Check sheet for the modelled part. Datum: model origin and axes. Units: mm. Face numbers are marked on the shaded views. A direction names the side the tool comes from. Coordinates: 2 decimals unless noted, no trailing zeros. Write each loop counter-clockwise with the first axis right and the second up, starting at its lowest first coordinate (ties: lowest second). Pieces come first, ordered by that corner, then holes. Notation, with made-up numbers: M -17,-16.5 L 13,-16.5 A11 ccw 13,3.5 Z; hole C 68.25,-10 d9. An arc over 180 degrees is marked long. Answer as CSV lines item,"result". Start each with the question number.
1) Draft check along Y on the marked faces 6, 7, 8 and 9. Enter one of: +Y half, -Y half, draft (parallel to the pull), parting line (faces both ways), or undercut.
2) Section check A-A (z = 12.5). Record the cut outline in (x, y), and give its area (3 significant figures).
3) Section check D-D (y = 38.25). Record the cut outline in (x, z).
4) Section check C-C (z = 15.75). Record the cut outline in (x, y).
5) Section check B-B (y = 50.25). Record the cut outline in (x, z), and give its area (3 significant figures).
6) Access from +Z, -Z, +X, -X, +Y, -Y to the whole of each face (thin tool, end or side, straight path). Record for the marked faces 1, 2, 3, 4 and 5.
7) Go/stop test with flat-tipped pins: pin 1 Ø6 at (x, y) = (-21.5, 54.5) entering from -Z; pin 2 Ø1.5 at (y, z) = (31.5, 19) entering from +X; pin 3 Ø6 at (x, y) = (-18.5, 10.5) entering from -Z. Record where each tip stops, or that it passes through.
8) Material ranges on L1, parallel to X at y = 38.25, z = 18.25; L2, parallel to X at y = 39, z = 24.25; L3, parallel to Y at x = -17, z = 19.75, recorded low to high. Write a range as [from, to].
from build123d import *

# Parameters (mm, degrees)
SKETCH_1_R          = 5
SKETCH_1_R_2        = 1.5
EXTRUDE_1_DEPTH     = 25
SKETCH_2_R          = 2.15
CUT_EXTRUDE_1_DEPTH = 30
SKETCH_3_R          = 2.15
CUT_EXTRUDE_2_DEPTH = 30
SKETCH_4_W          = 34
SKETCH_4_H          = 42.25
CUT_EXTRUDE_3_DEPTH = 15
CHAMFER_1_SIZE      = 5
CHAMFER_2_SIZE      = 3
SKETCH_6_R          = 9.75
CUT_EXTRUDE_5_DEPTH = 6.2
EXTRUDE_2_DEPTH     = 5
CHAMFER_3_SIZE      = 10


with BuildPart() as part:
    # 草图1 → 凸台-拉伸1 (new body)
    with BuildSketch(Plane.XY):
        Polygon((0, 0), (0, 20), (20, 20), (20, 25), (0, 25), (0, 67.25), (-34, 67.25), (-34, 20), (-5, 20), (-5, 0), align=None)
        with Locations((-17, 50.25)):
            Circle(SKETCH_1_R, mode=Mode.SUBTRACT)
        with Locations((-29, 62.25)):
            Circle(SKETCH_1_R_2, mode=Mode.SUBTRACT)
        with Locations((-5, 62.25)):
            Circle(SKETCH_1_R_2, mode=Mode.SUBTRACT)
        with Locations((-29, 38.25)):
            Circle(SKETCH_1_R_2, mode=Mode.SUBTRACT)
        with Locations((-5, 38.25)):
            Circle(SKETCH_1_R_2, mode=Mode.SUBTRACT)
    extrude(amount=EXTRUDE_1_DEPTH)

    # 草图2 → 切除-拉伸1 (cut)
    with BuildSketch(Plane(origin=(0, 0, 0), x_dir=(0, 0, -1), z_dir=(1, 0, 0))):
        with Locations((-12.5, 10)):
            Circle(SKETCH_2_R)
    extrude(amount=-CUT_EXTRUDE_1_DEPTH, mode=Mode.SUBTRACT)

    # 草图3 → 切除-拉伸2 (cut)
    with BuildSketch(Plane.XZ.offset(-20)):
        with Locations(Location((10, 12.5, 0), (0, 0, 270))):
            Circle(SKETCH_3_R)
    extrude(amount=-CUT_EXTRUDE_2_DEPTH, mode=Mode.SUBTRACT)

    # 草图4 → 切除-拉伸3 (cut)
    with BuildSketch(Plane(origin=(0, 0, 0), x_dir=(-1, 0, 0), z_dir=(0, 0, -1))):
        with Locations((17, 46.125)):
            Rectangle(SKETCH_4_W, SKETCH_4_H)
    extrude(amount=-CUT_EXTRUDE_3_DEPTH, mode=Mode.SUBTRACT)

    # 倒角1
    chamfer_1_edges = [part.edges().sort_by_distance(p)[0] for p in [
        (-5, 20, 12.5),
        (0, 25, 20),
    ]]
    chamfer(chamfer_1_edges, length=CHAMFER_1_SIZE)

    # 倒角2
    chamfer_2_edges = [part.edges().sort_by_distance(p)[0] for p in [
        (-34, 67.25, 20),
        (0, 67.25, 20),
    ]]
    chamfer(chamfer_2_edges, length=CHAMFER_2_SIZE)

    # 草图6 → 切除-拉伸5 (cut)
    with BuildSketch(Plane(origin=(0, 0, 15), x_dir=(-1, 0, 0), z_dir=(0, 0, -1))):
        with Locations((17, 50.25)):
            Circle(SKETCH_6_R)
    extrude(amount=-CUT_EXTRUDE_5_DEPTH, mode=Mode.SUBTRACT)

    # 草图7 → 凸台-拉伸2 (add)
    with BuildSketch(Plane.XY.offset(25)):
        Polygon((-34, 20), (-10, 20), (-5, 15), (-5, 0), align=None)
    extrude(amount=-EXTRUDE_2_DEPTH)

    # 倒角3
    # the kernel refuses this chamfer: 10 mm, written as the material it adds along each edge
    with BuildSketch(Plane(origin=(-34, 25, 15), x_dir=(0, 0.9996219169112968, 0.027495876610586317), z_dir=(1, 0, 0))) as chamfer_3_piece_1_section:
        Polygon((CHAMFER_3_SIZE * 0.999621916911, -CHAMFER_3_SIZE * 0.0274958766106), (-CHAMFER_3_SIZE * 0.0274958766106, -CHAMFER_3_SIZE * 0.999621916911), (0, 0), align=None)
    chamfer_3_piece_1 = extrude(amount=64.71682988, mode=Mode.PRIVATE)
    chamfer_3_piece_1 = split(chamfer_3_piece_1, bisect_by=Plane(origin=(0, 28.236246517, 11.669766102), z_dir=(-1, 0, 0)), keep=Keep.TOP, mode=Mode.PRIVATE)
    chamfer_3_piece_1 = split(chamfer_3_piece_1, bisect_by=Plane(origin=(-7.726936811, 37.726936811, 11.669766102), z_dir=(-0.7071067811865476, -0.7071067811865476, 0)), keep=Keep.TOP, mode=Mode.PRIVATE)
    add(chamfer_3_piece_1)
    with BuildSketch(Plane(origin=(-34, 25, 15), x_dir=(0, 0.9996219169112968, 0.027495876610586317), z_dir=(1, 0, 0))) as chamfer_3_piece_2_section:
        Polygon((CHAMFER_3_SIZE * 0.999621916911, -CHAMFER_3_SIZE * 0.0274958766106), (-CHAMFER_3_SIZE * 0.0274958766106, -CHAMFER_3_SIZE * 0.999621916911), (0, 0), align=None)
    chamfer_3_piece_2 = extrude(amount=64.71682988, mode=Mode.PRIVATE)
    chamfer_3_piece_2 = split(chamfer_3_piece_2, bisect_by=Plane(origin=(0, 26.323776193, 10.636124878), z_dir=(1, 0, 0)), keep=Keep.TOP, mode=Mode.PRIVATE)
    chamfer_3_piece_2 = split(chamfer_3_piece_2, bisect_by=Plane(origin=(2.757167855, 27.242832145, 10.636124878), z_dir=(-0.7071067811865476, -0.7071067811865476, 0)), keep=Keep.TOP, mode=Mode.PRIVATE)
    add(chamfer_3_piece_2)
    with BuildSketch(Plane(origin=(-34, 25, 15), x_dir=(0, 0.9996219169112968, 0.027495876610586317), z_dir=(1, 0, 0))) as chamfer_3_piece_3_section:
        Polygon((CHAMFER_3_SIZE * 0.999621916911, -CHAMFER_3_SIZE * 0.0274958766106), (-CHAMFER_3_SIZE * 0.0274958766106, -CHAMFER_3_SIZE * 0.999621916911), (0, 0), align=None)
    chamfer_3_piece_3 = extrude(amount=64.71682988, mode=Mode.PRIVATE)
    chamfer_3_piece_3 = split(chamfer_3_piece_3, bisect_by=Plane(origin=(0, 32.729927819, 14.022430088), z_dir=(-1, 0, 0)), keep=Keep.TOP, mode=Mode.PRIVATE)
    chamfer_3_piece_3 = split(chamfer_3_piece_3, bisect_by=Plane(origin=(-2.047445864, 32.047445864, 14.022430088), z_dir=(0.7071067811865476, 0.7071067811865476, 0)), keep=Keep.TOP, mode=Mode.PRIVATE)
    add(chamfer_3_piece_3)


solid = part.part
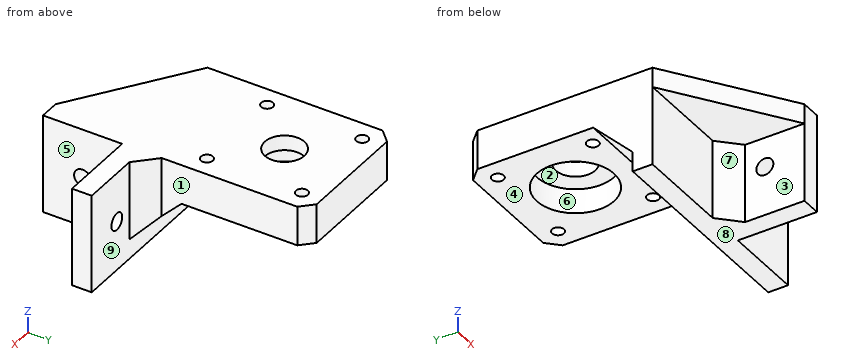
Results found:
1,face 6,"undercut"
1,face 7,"-Y half"
1,face 8,"draft"
1,face 9,"+Y half"
2,outline,"M -34,20 L -10,20 L -5,15 L -5,12.15 L 0,12.15 L 0,20 L 7.85,20 L 7.85,25 L 5,25 L 0,30 L 0,32.5 L -34,32.5 Z; M -5,0 L 0,0 L 0,7.85 L -5,7.85 Z; M 12.15,20 L 20,20 L 20,25 L 12.15,25 Z"
2,area,"607 mm2"
3,outline,"M -34,15 L -30.5,15 L -30.5,25 L -34,25 Z; M -27.5,15 L -6.5,15 L -6.5,25 L -27.5,25 Z; M -3.5,15 L 0,15 L 0,25 L -3.5,25 Z"
4,outline,"M -34,20 L -10,20 L -5,15 L -5,0 L 0,0 L 0,20 L 20,20 L 20,25 L 5,25 L 0,30 L 0,64.25 L -3,67.25 L -31,67.25 L -34,64.25 Z; hole C -29,38.25 d3; hole C -29,62.25 d3; hole C -17,50.25 d19.5; hole C -5,38.25 d3; hole C -5,62.25 d3"
5,outline,"M -34,15 L -26.75,15 L -26.75,21.2 L -22,21.2 L -22,25 L -34,25 Z; M -12,21.2 L -7.25,21.2 L -7.25,15 L 0,15 L 0,25 L -12,25 Z"
5,area,"181 mm2"
6,face 1,"+Z, -Z, +X, +Y"
6,face 2,"-Z"
6,face 3,"-Z, -X, -Y"
6,face 4,"-Z, +X, -X, +Y"
6,face 5,"+Z, -Z, +X, -Y"
7,pin 1,"stops at z = 21.2"
7,pin 2,"stops at x = 0"
7,pin 3,"stops at z = 20"
8,L1,"x = [-34, -30.5], [-27.5, -6.5], [-3.5, 0]"
8,L2,"x = [-34, -30.3], [-27.7, -6.3], [-3.7, 0]"
8,L3,"y = [20, 40.5], [60, 67.25]"
